Could you check a few things on this model? Use its own coordinates, in mm. A direction names the side the tool comes from. Round coordinates to 2 decimals unless told otherwise and drop trailing zeros. Loops run counter-clockwise (first coordinate to the right, second up) from the corner with the lowest first, then second, coordinate; pieces in that order, holes last. Notation, with made-up numbers: (78, 45.5) -> (114, 45.5) arc R8 ccw to (114, 59.5) -> close; hole circle Ø11 at (-29.75, 14.5). An arc over 180 degrees is marked (long way). Write each question's results on one line, items separated by ' | '. Start each with the question number.
1) If I drill on probe 1 along Z at (x, y) = (-5, -8); probe 2 along Z at (x, y) = (3, -4.5); probe 3 along Y at (x, z) = (7.5, 44), over which ranges is the centre line in solid material (lowest first)?
2) Imagine slicing it at C-C, the plane z = 25. List the corners of the cut face in (x, y) for me, plus the area to 3 significant figures.
3) We'd pull the mould along Y, two halves only. Please class faces 1 (the cylindrical face through (7.595, 10.124, 43.479)), 2 (the flat face through (-15, 3, 45)), 3 (the cylindrical face through (8.816, 4.871, 43.479)), 4 (the cylindrical face through (-0.54, -2.44, 58.86)): pulls with the +Y half, pulls with the -Y half, needs draft (parallel to the pull), parting line crosses it, or undercut.
4) Imagine slicing it at B-B, the plane y = -13. List the corners of the cut face in (x, z) for me, plus the area to 3 significant figures.
5) Imagine slicing it at A-A, the plane x = 0. List the corners of the cut face in (y, z) for me.
6) Imagine slicing it at D-D, the plane z = 47.5. List the corners of the cut face in (x, y) for me, plus the area to 3 significant figures.
7) Which directions (+Z, -Z, +X, -X, +Y, -Y) give clear straight access to the entire face, cutting with the end or side of a thin tool? Please do faces 5 (the flat face through (-15, -3, 45)), 6 (the flat face through (-2, -2, 49)), 7 (the cylindrical face through (3.68, -8.99, 45.45)), 8 (the flat face through (6, 12, 45)).
8) For P1, Ø1.5, axis at x = -2.5, z = 26.5, coming from the +Y side; P2, Ø8, axis at x = -4, y = -10.5, coming from the +Z side; P3, Ø2, axis at x = -2, y = 2, coming from the +Z side; P4, Ø2.5, axis at x = 6, y = 12.5, coming from the +Z side, each with a flat end and sliding along its axis, tell me the tip position at first contact or that it passes through.
from build123d import *

# Parameters (mm, degrees)
F0_R     = 18.5
F1_DEPTH = 42
F3_DEPTH = 7
F4_R     = 2.54
F5_R     = 2.5
F6_DEPTH = 20
F8_R     = 1.5
F7_R     = 1.5
F9_DEPTH = 3


with BuildPart() as f1:
    # F0 (on Top) → F1 (new body)
    with BuildSketch(Plane.XY):
        Circle(F0_R)
    extrude(amount=F1_DEPTH)

    # F2 (on face) → F3 (join)
    with BuildSketch(Plane.XY.offset(42)):
        with BuildLine():
            ThreePointArc((-18.2551362635, 3), (-18.5, 0), (-18.2551362635, -3))
            Line((-18.2551362635, -3), (-12.357306623, -3))
            ThreePointArc((-12.357306623, -3), (-9.5173301957, -3.5232332201), (-7.0502937278, -5.0242229525))
            Line((-7.0502937278, -5.0242229525), (-5.6619374598, -6.2636447322))
            ThreePointArc((-5.6619374598, -6.2636447322), (-3.695866688, -8.9516216481), (-3, -12.2083721348))
            Line((-3, -12.2083721348), (-3, -18.2551362635))
            ThreePointArc((-3, -18.2551362635), (0, -18.5), (3, -18.2551362635))
            Line((3, -18.2551362635), (3, -12.2083721348))
            ThreePointArc((3, -12.2083721348), (3.695866688, -8.9516216481), (5.6619374598, -6.2636447322))
            Line((5.6619374598, -6.2636447322), (7.0502937278, -5.0242229525))
            ThreePointArc((7.0502937278, -5.0242229525), (9.5173301957, -3.5232332201), (12.357306623, -3))
            Line((12.357306623, -3), (18.2551362635, -3))
            ThreePointArc((18.2551362635, -3), (18.4386824485, -1.5049882267), (18.5, 0))
            ThreePointArc((18.5, 0), (18.4386824485, 1.5049882267), (18.2551362635, 3))
            Line((18.2551362635, 3), (12.357306623, 3))
            ThreePointArc((12.357306623, 3), (9.5173301957, 3.5232332201), (7.0502937278, 5.0242229525))
            Line((7.0502937278, 5.0242229525), (5.6619374598, 6.2636447322))
            ThreePointArc((5.6619374598, 6.2636447322), (3.695866688, 8.9516216481), (3, 12.2083721348))
            Line((3, 12.2083721348), (3, 18.2551362635))
            ThreePointArc((3, 18.2551362635), (0, 18.5), (-3, 18.2551362635))
            Line((-3, 18.2551362635), (-3, 12.2083721348))
            ThreePointArc((-3, 12.2083721348), (-3.695866688, 8.9516216481), (-5.6619374598, 6.2636447322))
            Line((-5.6619374598, 6.2636447322), (-7.0502937278, 5.0242229525))
            ThreePointArc((-7.0502937278, 5.0242229525), (-9.5173301957, 3.5232332201), (-12.357306623, 3))
            Line((-12.357306623, 3), (-18.2551362635, 3))
        make_face()
    extrude(amount=F3_DEPTH)

    # F4
    f4_edges = [f1.edges().sort_by_distance(p)[0] for p in [
        (0, 18.5, 49),
        (-18.5, 0, 49),
        (0, -18.5, 49),
        (18.5, 0, 49),
    ]]
    fillet(f4_edges, radius=F4_R)

    # F5 (on face) → F6 (join)
    with BuildSketch(Plane.XY.offset(49)):
        Circle(F5_R)
    extrude(amount=F6_DEPTH)

    # F8 (on face) + F7 (on face) → F9 (join)
    with BuildSketch(Plane.XY.offset(42)):
        with Locations((6.1871920723, 11.9740978757)):
            Circle(F8_R)
    with BuildSketch(Plane.XY.offset(42)):
        with Locations((7.7906422209, 8.6364694748)):
            Circle(F7_R)
        with Locations((10.0058761309, 5.7833763727)):
            Circle(F7_R)
    extrude(amount=F9_DEPTH)


solid = f1.part
Checked values:
1) probe 1: 0 to 42 | probe 2: 0 to 49 | probe 3: -4.65 to 4.65, 7.16 to 10.11, 11.25 to 12.7
2) outline: circle Ø37 at (0, 0) | area: 1,080 mm^2
3) face 1: undercut | face 2: pulls with the +Y half | face 3: undercut | face 4: parting line crosses it
4) outline: (-13.16, 0) -> (13.16, 0) -> (13.16, 42) -> (3, 42) -> (3, 49) -> (-3, 49) -> (-3, 42) -> (-13.16, 42) -> close | area: 1,150 mm^2
5) outline: (-18.5, 0) -> (18.5, 0) -> (18.5, 46.46) arc R2.54 ccw to (15.96, 49) -> (2.5, 49) -> (2.5, 69) -> (-2.5, 69) -> (-2.5, 49) -> (-15.96, 49) arc R2.54 ccw to (-18.5, 46.46) -> close
6) outline: (-18.03, -3) -> (-12.36, -3) arc R7.97 cw to (-7.05, -5.02) -> (-5.66, -6.26) arc R7.97 cw to (-3, -12.21) -> (-3, -18.03) arc R18.28 ccw to (3, -18.03) -> (3, -12.21) arc R7.97 cw to (5.66, -6.26) -> (7.05, -5.02) arc R7.97 cw to (12.36, -3) -> (18.03, -3) arc R18.28 ccw to (18.03, 3) -> (12.36, 3) arc R7.97 cw to (7.05, 5.02) -> (5.66, 6.26) arc R7.97 cw to (3, 12.21) -> (3, 18.03) arc R18.28 ccw to (-3, 18.03) -> (-3, 12.21) arc R7.97 cw to (-5.66, 6.26) -> (-7.05, 5.02) arc R7.97 cw to (-12.36, 3) -> (-18.03, 3) arc R18.28 ccw to start | area: 483 mm^2
7) face 5: +Z, -X, -Y | face 6: +Z | face 7: +Z, +X, -Y | face 8: +Z, +X, +Y
8) P1: y = 18.42 | P2: z = 49 | P3: z = 69 | P4: z = 45
